Geometry check sheet. Reference: the model listing, model coordinates, mm. Coordinates: 2 decimals unless noted, no trailing zeros. Loops run counter-clockwise (first coordinate to the right, second up) from the corner with the lowest first, then second, coordinate; pieces in that order, holes last. Notation, with made-up numbers: (88, 12.5) -> (140, 12.5) arc R31 ccw to (140, 47.5) -> close; hole circle Ø4 at (77.5, 46). An arc over 180 degrees is marked (long way). Answer as a JSON object with one key per item and string values.
from build123d import *

# Parameters (mm, degrees)
SKETCH_2_W      = 25.0000008
SKETCH_2_H      = 15.04999784
EXTRUDE_2_DEPTH = 24
SKETCH_3_R      = 0.5
EXTRUDE_3_DEPTH = 5
SKETCH_4_W      = 2.5
SKETCH_4_H      = 7
EXTRUDE_4_DEPTH = 2


with BuildPart() as part:
    # Эскиз2 → Бобышка-Вытянуть2 (new body)
    with BuildSketch(Plane.XY):
        with Locations((-17.07912528, 17.543231945)):
            Rectangle(SKETCH_2_W, SKETCH_2_H)
    extrude(amount=EXTRUDE_2_DEPTH)

    # Эскиз3 → Бобышка-Вытянуть3 (add)
    with BuildSketch(Plane(origin=(0, 0, 0), x_dir=(-1, 0, 0), z_dir=(0, 0, -1))):
        with Locations(Location((24.67912568, 20.568230865, 0), (0, 0, 180))):
            Circle(SKETCH_3_R)
        with Locations(Location((24.67912568, 14.568230865, 0), (0, 0, 180))):
            Circle(SKETCH_3_R)
    extrude(amount=EXTRUDE_3_DEPTH)

    # Эскиз4 → Бобышка-Вытянуть4 (add)
    with BuildSketch(Plane(origin=(0, 0, 0), x_dir=(-1, 0, 0), z_dir=(0, 0, -1))):
        with Locations((17.07912488, 25.568230865)):
            Rectangle(SKETCH_4_W, SKETCH_4_H)
        with Locations((17.07912488, 9.518233025)):
            Rectangle(SKETCH_4_W, SKETCH_4_H)
    extrude(amount=EXTRUDE_4_DEPTH)


solid = part.part
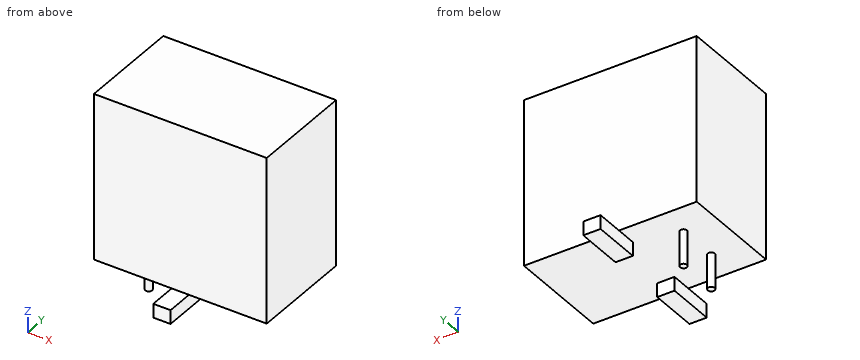
1. Depth check by flat-ended pin: P1, Ø7, axis at x = -15, z = 7.5, coming from the +Y side; P2, Ø3, axis at x = -17, y = 28, coming from the +Z side; P3, Ø2, axis at y = 8, z = -1, coming from the +X side. Enter the tip coordinate at first touch or a pass-through.
Evaluation:
{"P1": "stops at y = 25.07", "P2": "stops at z = 0", "P3": "stops at x = -15.83"}
2. Section check A-A, the plane z = -0.75. Record the boundary of the cut face in (x, y), then the cut area to 3 significant figures.
Evaluation:
{"outline": "circle Ø1 at (-24.68, 14.57); circle Ø1 at (-24.68, 20.57); (-18.33, 6.02) -> (-15.83, 6.02) -> (-15.83, 13.02) -> (-18.33, 13.02) -> close; (-18.33, 22.07) -> (-15.83, 22.07) -> (-15.83, 29.07) -> (-18.33, 29.07) -> close", "area": "36.6 mm^2"}
3. Section check D-D, the plane z = 17.75. Record the boundary of the cut face in (x, y), then the cut area to 3 significant figures.
Evaluation:
{"outline": "(-29.58, 10.02) -> (-4.58, 10.02) -> (-4.58, 25.07) -> (-29.58, 25.07) -> close", "area": "376 mm^2"}
4. Section check C-C, the plane x = -12.75. Record the boundary of the cut face in (y, z), then the cut area to 3 significant figures.
Evaluation:
{"outline": "(10.02, 0) -> (25.07, 0) -> (25.07, 24) -> (10.02, 24) -> close", "area": "361 mm^2"}
5. Section check B-B, the plane y = 11.25. Record the boundary of the cut face in (x, z).
Evaluation:
{"outline": "(-29.58, 0) -> (-18.33, 0) -> (-18.33, -2) -> (-15.83, -2) -> (-15.83, 0) -> (-4.58, 0) -> (-4.58, 24) -> (-29.58, 24) -> close"}
6. Thickness scan on probe 1 along Y at (x, z) = (-11.5, 5.5); probe 2 along X at (y, z) = (9.5, -0.25); probe 3 along Z at (x, y) = (-20, 21.25). Record the ranges inside material, lowest first. Write a range as from..to.
Evaluation:
{"probe 1": "y = 10.02..25.07", "probe 2": "x = -18.33..-15.83", "probe 3": "z = 0..24"}
